Read the model definition and answer for the solid it produces. Units are mm, in the model's axes. A direction names the side the tool comes from. Coordinates: 2 decimals unless noted, no trailing zeros. Loops run counter-clockwise (first coordinate to the right, second up) from the corner with the lowest first, then second, coordinate; pieces in that order, holes last. Notation, with made-up numbers: (-7, 57.5) - (52, 57.5) arc R21 ccw to (52, 91.5) - close; hole circle Ø10 at (12, 78). An arc over 180 degrees is marked (long way). Use CSV: the item, a comma, the result in double quotes.
```python
from build123d import *

# Parameters (mm, degrees)
F0_R     = 30
F0_R_2   = 8.5
F1_DEPTH = 2.5
F3_DEPTH = 37
F4_DEPTH = 40


with BuildPart() as f1:
    # F0 (on Front) → F1 (new body)
    with BuildSketch(Plane.XZ):
        Circle(F0_R)
        Circle(F0_R_2, mode=Mode.SUBTRACT)
    extrude(amount=-F1_DEPTH)

    # F2 (on Front) → F3 (join)
    with BuildSketch(Plane.XZ):
        with BuildLine():
            ThreePointArc((9.9539621754, -0.9584555339), (9.9884839128, -0.4797802861), (10, 0))
            ThreePointArc((10, 0), (9.9474412154, 1.0239205366), (9.790317347, 2.0370778693))
            ThreePointArc((9.790317347, 2.0370778693), (9.0162927853, 4.3250970404), (7.7162445614, 6.3607837464))
            ThreePointArc((7.7162445614, 6.3607837464), (6.6748253827, 7.4462545021), (5.4823682108, 8.3632313612))
            ThreePointArc((5.4823682108, 8.3632313612), (3.3171763231, 9.4337872163), (0.9584555339, 9.9539621754))
            ThreePointArc((0.9584555339, 9.9539621754), (-0.5454827615, 9.9851113442), (-2.0370778693, 9.790317347))
            ThreePointArc((-2.0370778693, 9.790317347), (-4.3250970404, 9.0162927853), (-6.3607837464, 7.7162445614))
            ThreePointArc((-6.3607837464, 7.7162445614), (-7.4462545021, 6.6748253827), (-8.3632313612, 5.4823682108))
            ThreePointArc((-8.3632313612, 5.4823682108), (-9.4337872163, 3.3171763231), (-9.9539621754, 0.9584555339))
            ThreePointArc((-9.9539621754, 0.9584555339), (-9.9851113442, -0.5454827615), (-9.790317347, -2.0370778693))
            ThreePointArc((-9.790317347, -2.0370778693), (-9.0162927853, -4.3250970404), (-7.7162445614, -6.3607837464))
            ThreePointArc((-7.7162445614, -6.3607837464), (-6.6748253827, -7.4462545021), (-5.4823682108, -8.3632313612))
            ThreePointArc((-5.4823682108, -8.3632313612), (-3.3171763231, -9.4337872163), (-0.9584555339, -9.9539621754))
            ThreePointArc((-0.9584555339, -9.9539621754), (0.5454827615, -9.9851113442), (2.0370778693, -9.790317347))
            ThreePointArc((2.0370778693, -9.790317347), (4.3250970404, -9.0162927853), (6.3607837464, -7.7162445614))
            ThreePointArc((6.3607837464, -7.7162445614), (7.4462545021, -6.6748253827), (8.3632313612, -5.4823682108))
            ThreePointArc((8.3632313612, -5.4823682108), (9.4337872163, -3.3171763231), (9.9539621754, -0.9584555339))
        make_face()
        with BuildLine():
            ThreePointArc((-8.3632313612, 5.4823682108), (-7.4462545021, 6.6748253827), (-6.3607837464, 7.7162445614))
            Line((-6.3607837464, 7.7162445614), (-17.9943087682, 17.355254304))
            ThreePointArc((-17.9943087682, 17.355254304), (-19.0032050673, 16.2443281539), (-19.9436281467, 15.0748696959))
            Line((-19.9436281467, 15.0748696959), (-8.3632313612, 5.4823682108))
        make_face()
        with BuildLine():
            Line((-15.0748696959, -19.9436281467), (-5.4823682108, -8.3632313612))
            ThreePointArc((-5.4823682108, -8.3632313612), (-6.6748253827, -7.4462545021), (-7.7162445614, -6.3607837464))
            Line((-7.7162445614, -6.3607837464), (-17.355254304, -17.9943087682))
            ThreePointArc((-17.355254304, -17.9943087682), (-16.2443281539, -19.0032050673), (-15.0748696959, -19.9436281467))
        make_face()
        with BuildLine():
            Line((3.4427321165, -24.7618172914), (2.0370778693, -9.790317347))
            ThreePointArc((2.0370778693, -9.790317347), (0.5454827615, -9.9851113442), (-0.9584555339, -9.9539621754))
            Line((-0.9584555339, -9.9539621754), (0.4518797452, -24.9959157603))
            ThreePointArc((0.4518797452, -24.9959157603), (1.9508205739, -24.9237697608), (3.4427321165, -24.7618172914))
        make_face()
        with BuildLine():
            Line((19.9436281467, -15.0748696959), (8.3632313612, -5.4823682108))
            ThreePointArc((8.3632313612, -5.4823682108), (7.4462545021, -6.6748253827), (6.3607837464, -7.7162445614))
            Line((6.3607837464, -7.7162445614), (17.9943087682, -17.355254304))
            ThreePointArc((17.9943087682, -17.355254304), (19.0032050673, -16.2443281539), (19.9436281467, -15.0748696959))
        make_face()
        with BuildLine():
            ThreePointArc((9.790317347, 2.0370778693), (9.9474412154, 1.0239205366), (10, 0))
            ThreePointArc((10, 0), (9.9884839128, -0.4797802861), (9.9539621754, -0.9584555339))
            Line((9.9539621754, -0.9584555339), (24.9959157603, 0.4518797452))
            ThreePointArc((24.9959157603, 0.4518797452), (24.9237697608, 1.9508205739), (24.7618172914, 3.4427321165))
            Line((24.7618172914, 3.4427321165), (9.790317347, 2.0370778693))
        make_face()
        with BuildLine():
            ThreePointArc((5.4823682108, 8.3632313612), (6.6748253827, 7.4462545021), (7.7162445614, 6.3607837464))
            Line((7.7162445614, 6.3607837464), (17.355254304, 17.9943087682))
            ThreePointArc((17.355254304, 17.9943087682), (16.2443281539, 19.0032050673), (15.0748696959, 19.9436281467))
            Line((15.0748696959, 19.9436281467), (5.4823682108, 8.3632313612))
        make_face()
        with BuildLine():
            ThreePointArc((-2.0370778693, 9.790317347), (-0.5454827615, 9.9851113442), (0.9584555339, 9.9539621754))
            Line((0.9584555339, 9.9539621754), (-0.4518797452, 24.9959157603))
            ThreePointArc((-0.4518797452, 24.9959157603), (-1.9508205739, 24.9237697608), (-3.4427321165, 24.7618172914))
            Line((-3.4427321165, 24.7618172914), (-2.0370778693, 9.790317347))
        make_face()
        with BuildLine():
            ThreePointArc((-9.790317347, -2.0370778693), (-9.9851113442, -0.5454827615), (-9.9539621754, 0.9584555339))
            Line((-9.9539621754, 0.9584555339), (-24.9959157603, -0.4518797452))
            ThreePointArc((-24.9959157603, -0.4518797452), (-24.9237697608, -1.9508205739), (-24.7618172914, -3.4427321165))
            Line((-24.7618172914, -3.4427321165), (-9.790317347, -2.0370778693))
        make_face()
    extrude(amount=F3_DEPTH)

    # F4 (cut): a face of the model
    f4_faces = [f1.faces().sort_by_distance(p)[0] for p in [
        (0, 0, 0),
    ]]
    extrude(f4_faces, amount=-F4_DEPTH, mode=Mode.SUBTRACT)


solid = f1.part
```
Q1. For a pull along X with two mould halves and no side action, classify faces 6 (the face through (-16.26, -18.24, -18.99)), 7 (the face through (0.263, -18.241, 17.37)), 8 (the face through (-29.97, 1.23, 1.32)), 9 (the face through (2.75, -18.24, -17.38)) as +X half, -X half, draft (parallel to the pull), parting line (faces both ways), or undercut.
Reported:
face 6,"-X half"
face 7,"undercut"
face 8,"parting line"
face 9,"undercut"
Q2. The part is cut by section C-C on z = -21.5. Determine the outline of the cut face in (x, y).
Reported:
outline,"(-20.92, 0) - (0.12, 0) - (0.12, -37) - (3.14, -37) - (3.14, 0) - (20.92, 0) - (20.92, 2.5) - (-20.92, 2.5) - close"
Q3. A tool of negligible diameter and unlimited length cuts with its end or side. For faces 1 (the face through (9.422, -18.241, -3.349)), 2 (the face through (18.99, -18.24, -16.26)), 3 (the face through (6, 0, -13)), 4 (the face through (-17.37, -18.241, 0.263)), 5 (the face through (12.1, -18.24, -12.47)), from which of +Z, -Z, +X, -X, +Y, -Y can it reach the whole face along a straight path? Write none if from no direction.
Reported:
face 1,"+X, -Y"
face 2,"-Z, +X, -Y"
face 3,"-Y"
face 4,"-X, -Y"
face 5,"-Z, -Y"
Q4. Find the intervals of material crossed by probe 1 along X at (y, z) = (-10.5, -16); probe 2 along X at (y, z) = (-5.5, 15); probe 3 along Y at (x, z) = (-15.5, 15.5), in increasing order. Write a range as [from, to].
Reported:
probe 1,"x = [-15.7, -11.81], [-0.39, 2.62], [16.36, 19.21]"
probe 2,"x = [-19.85, -15.15], [-2.53, 0.49], [10.98, 14.87]"
probe 3,"y = [0, 2.5]"
Q5. The part is cut by section D-D on x = 16. Determine the outline of the cut face in (y, z), and give its area (3 significant figures).
Reported:
outline,"(-37, -15.7) - (0, -15.7) - (0, -25.38) - (2.5, -25.38) - (2.5, 25.38) - (0, 25.38) - (0, 19.21) - (-37, 19.21) - (-37, 16.36) - (0, 16.36) - (0, 2.62) - (-37, 2.62) - (-37, -0.39) - (0, -0.39) - (0, -11.81) - (-37, -11.81) - close"
area,"488 mm²"
Q6. The part is cut by section B-B on x = 4.5. Determine the outline of the cut face in (y, z), and give its area (3 significant figures).
Reported:
outline,"(-37, -8.93) - (0, -8.93) - (0, -29.66) - (2.5, -29.66) - (2.5, -7.21) - (-37, -7.21) - close; (-37, 7.21) - (2.5, 7.21) - (2.5, 29.66) - (0, 29.66) - (0, 8.93) - (-37, 8.93) - close"
area,"239 mm²"
Q7. Given P1, Ø2, axis at x = 0, y = -10, coming from the -Z side; P2, Ø5, axis at y = -13.5, z = -19.5, coming from the -X side; P3, Ø1, axis at x = 5.5, y = -22.5, coming from the +Z side, each flat-ended and moving along its own axis, determine where each tip first touches the part or whether it passes through.
Reported:
P1,"stops at z = -25"
P2,"stops at x = -17.36"
P3,"stops at z = 8.99"
